Read the model definition and answer for the solid it produces. Units are mm, in the model's axes. Face numbers are marked on the shaded views. Coordinates: 2 decimals unless noted, no trailing zeros. Write each loop counter-clockwise with the first axis right and the second up, starting at its lowest first coordinate (ties: lowest second). Pieces come first, ordered by that corner, then holes.
(1) Given pin 1 (5.5 mm diameter, centred on x = -2.5, z = 2.5, fed in from -Y); pin 2 (1 mm diameter, centred on y = 15.5, z = 0.5, fed in from +X); pin 3 (1.5 mm diameter, centred on x = -6.5, y = 17, fed in from +Z), each flat-ended and moving along its own axis, determine where each tip first touches the part or whether it passes through.
(2) Straight lines are drawn through the part: line 1 along Z through (x, y) = (0, 5.25); line 2 along Y through (x, z) = (2, 2); line 3 along Z through (x, y) = (8, 6.35). For each, find the intervals that lie inside material, in ascending order.
(3) The part is cut by section B-B, the plane y = 8.5. Determine the outline of the cut face in (x, z).
(4) The part is cut by section C-C, the plane y = 36. Determine the outline of the cut face in (x, z).
(5) The part is cut by section A-A, the plane y = 21. Determine the outline of the cut face in (x, z), and give its area (3 significant figures).
(6) Determine the mould class of the marked faces 1, 2, 3 and 4 for opening direction Z: pulls with the +Z half, pulls with the -Z half, needs draft (parallel to the pull), parting line crosses it, or undercut.
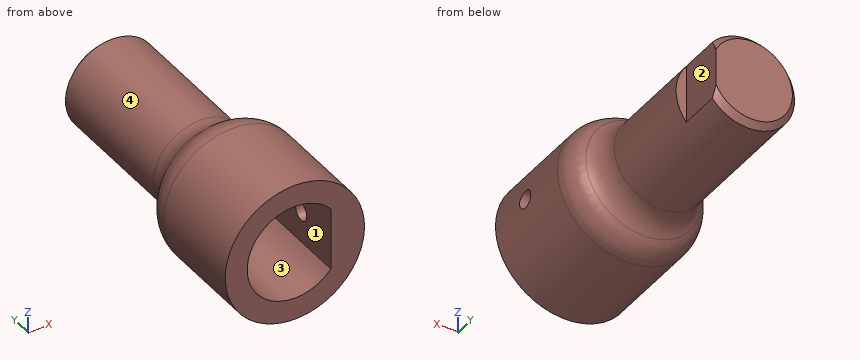
```python
from build123d import *

# Parameters (mm, degrees)
SKETCH1_R           = 6.2865
BASE_EXTRUDE_DEPTH  = 40
SKETCH3_R           = 9.4615
BOSS_EXTRUDE1_DEPTH = 15.875
CUT_EXTRUDE1_DEPTH  = 12.7
FILLET1_R           = 4.7625
FILLET2_R           = 4.7625
SKETCH5_R           = 1.190625
CUT_EXTRUDE2_DEPTH  = 44.537009406
CUT_EXTRUDE3_START  = -6.35
CUT_EXTRUDE3_DEPTH  = 6.35
CHAMFER1_SIZE       = 0.79375


with BuildPart() as part:
    # Sketch1 → Base-Extrude (new body)
    with BuildSketch(Plane(origin=(0, 0, 0), x_dir=(-1, 0, 0), z_dir=(0, 1, 0))):
        with Locations(Location((0, 0, 0), (0, 0, 90))):
            Circle(SKETCH1_R)
    extrude(amount=BASE_EXTRUDE_DEPTH)

    # Sketch3 → Boss-Extrude1 (add)
    with BuildSketch(Plane(origin=(0, 0, 0), x_dir=(-1, 0, 0), z_dir=(0, 1, 0))):
        with Locations(Location((0, 0, 0), (0, 0, 90))):
            Circle(SKETCH3_R)
    extrude(amount=BOSS_EXTRUDE1_DEPTH)

    # Sketch4 → Cut-Extrude1 (cut)
    with BuildSketch(Plane(origin=(0, 0, 0), x_dir=(-1, 0, 0), z_dir=(0, 1, 0))):
        with BuildLine():
            Line((-4.8895, 4.247860491), (-4.8895, -4.247860491))
            ThreePointArc((-4.8895, -4.247860491), (6.477, 0), (-4.8895, 4.247860491))
        make_face()
    extrude(amount=CUT_EXTRUDE1_DEPTH, mode=Mode.SUBTRACT)

    # Fillet1
    # the kernel refuses this fillet: 4.7625 mm, written as the material it adds along each edge
    with BuildSketch(Plane(origin=(0, 15.875, 0), x_dir=(0, 0, 1), z_dir=(1, 0, 0))) as fillet1_piece_1:
        with BuildLine():
            CenterArc((11.049, -4.490128061), FILLET1_R, 109.471220634, 70.528779366)
            Line((6.2865, -4.490128061), (6.19125, -4.490128061))
            Line((6.19125, -4.490128061), (6.19125, 0))
            Line((6.19125, 0), (6.2865, 0.09525))
            ThreePointArc((6.2865, 0.09525), (7.874, 0.09525), (9.42975, 0.089802561))
            Line((9.42975, 0.089802561), (9.4615, 0))
        make_face()
    revolve(axis=Axis((0, 15.875, 0), (0, -1, 0)))

    # Fillet2
    fillet2_edges = [part.edges().sort_by_distance(p)[0] for p in [
        (0, 15.875, -9.4615),
    ]]
    fillet(fillet2_edges, radius=FILLET2_R)

    # Sketch5 → Cut-Extrude2 (cut, through all)
    with BuildSketch(Plane.ZY.offset(-4.8895)):
        with Locations((0, 6.35)):
            Circle(SKETCH5_R)
    extrude(amount=-CUT_EXTRUDE2_DEPTH, mode=Mode.SUBTRACT)

    # Sketch7 → Cut-Extrude3 (cut)
    with BuildSketch(Plane(origin=(0, 40, 0), x_dir=(-1, 0, 0), z_dir=(0, 1, 0)).offset(CUT_EXTRUDE3_START)):
        with BuildLine():
            Line((-4.8895, 3.951312693), (-4.8895, -3.951312693))
            ThreePointArc((-4.8895, -3.951312693), (-6.2865, 0), (-4.8895, 3.951312693))
        make_face()
    extrude(amount=CUT_EXTRUDE3_DEPTH, mode=Mode.SUBTRACT)

    # Chamfer1
    chamfer1_edges = [part.edges().sort_by_distance(p)[0] for p in [
        (-5.67274226, 40, -2.70925774),
    ]]
    chamfer(chamfer1_edges, length=CHAMFER1_SIZE)


solid = part.part
```
Computed:
1. pin 1: stops at y = 12.7
1. pin 2: stops at x = 9.12
1. pin 3: stops at z = 5.66
2. line 1: z = -9.46 to -6.48, 6.48 to 9.46
2. line 2: y = 12.7 to 40
2. line 3: z = -5.05 to -1.19, 1.19 to 5.05
3. outline: circle Ø18.92 at (0, 0); hole (4.89, -4.25) - (4.89, 4.25) arc R6.48 ccw (long way) to start
4. outline: (4.89, -3.95) - (4.89, 3.95) arc R6.29 ccw (long way) to start
5. outline: circle Ø12.57 at (0, 0)
5. area: 124 mm2
6. face 1: undercut
6. face 2: needs draft
6. face 3: undercut
6. face 4: parting line crosses it
